The listing builds one solid part. Answer for the finished solid, in the listing's coordinates (mm). A direction names the side the tool comes from. Coordinates: 2 decimals unless noted, no trailing zeros. Write each loop counter-clockwise with the first axis right and the second up, starting at its lowest first coordinate (ties: lowest second). Pieces come first, ordered by that corner, then holes.
from build123d import *

# Parameters (mm, degrees)
SKETCH1_W           = 106
SKETCH1_H           = 48
SKETCH1_R           = 2.5
BOSS_EXTRUDE3_DEPTH = 3
BOSS_EXTRUDE4_DEPTH = 24


with BuildPart() as part:
    # Sketch1 → Boss-Extrude3 (new body)
    with BuildSketch(Plane(origin=(0, 0, 0), x_dir=(1, 0, 0), z_dir=(0, 1, 0))):
        with Locations((-8.19327026, 12.513208654)):
            Rectangle(SKETCH1_W, SKETCH1_H)
        with Locations(Location((-54.723551999, 30.013208654, 0), (0, 0, 270))):
            Circle(SKETCH1_R, mode=Mode.SUBTRACT)
        with Locations(Location((-54.690171501, -4.986791346, 0), (0, 0, 270))):
            Circle(SKETCH1_R, mode=Mode.SUBTRACT)
        with Locations(Location((38.31560417, 30.013208654, 0), (0, 0, 270))):
            Circle(SKETCH1_R, mode=Mode.SUBTRACT)
        with Locations(Location((38.297946807, -4.986791346, 0), (0, 0, 270))):
            Circle(SKETCH1_R, mode=Mode.SUBTRACT)
    extrude(amount=BOSS_EXTRUDE3_DEPTH)

    # Sketch3 → Boss-Extrude4 (add)
    with BuildSketch(Plane(origin=(0, 3, 0), x_dir=(1, 0, 0), z_dir=(0, 1, 0))):
        Polygon((-44.19327026, 32.513208654), (-44.19327026, -7.486791346), (-21.19327026, -7.486791346), (-21.19327026, -11.486791346), (-48.19327026, -11.486791346), (-48.19327026, 36.513208654), (31.80672974, 36.513208654), (31.80672974, -11.486791346), (4.80672974, -11.486791346), (4.80672974, -7.486791346), (27.80672974, -7.486791346), (27.80672974, 32.513208654), align=None)
    extrude(amount=BOSS_EXTRUDE4_DEPTH)


solid = part.part
1. Section C-C on x = -11.5 is taken. Give the vertices of the cut face in (y, z).
Results found:
outline: (0, -36.51) - (27, -36.51) - (27, -32.51) - (3, -32.51) - (3, 11.49) - (0, 11.49) - close
2. For a pull along X with two mould halves and no side action, classify faces 6 (the flat face through (-9, 1, 11.487)), 7 (the flat face through (-61.193, 1, -12)), 8 (the flat face through (-9, 3, -11)) as pulls with the +X half, pulls with the -X half, needs draft (parallel to the pull), parting line crosses it, or undercut.
Results found:
face 6: needs draft
face 7: pulls with the -X half
face 8: undercut
3. Find the intervals of material crossed by L1, parallel to X at y = 12, z = -15.5; L2, parallel to Z at x = -24, y = 22; L3, parallel to Y at x = 34, z = -5.5, in increasing order.
Results found:
L1: x = -48.19 to -44.19, 27.81 to 31.81
L2: z = -36.51 to -32.51, 7.49 to 11.49
L3: y = 0 to 3
4. Section B-B on y = 21 is taken. Give the vertices of the cut face in (x, z).
Results found:
outline: (-48.19, -36.51) - (31.81, -36.51) - (31.81, 11.49) - (4.81, 11.49) - (4.81, 7.49) - (27.81, 7.49) - (27.81, -32.51) - (-44.19, -32.51) - (-44.19, 7.49) - (-21.19, 7.49) - (-21.19, 11.49) - (-48.19, 11.49) - close
5. Section D-D on x = 7 is taken. Give the vertices of the cut face in (y, z), then the cut area to 3 significant figures.
Results found:
outline: (0, -36.51) - (27, -36.51) - (27, -32.51) - (3, -32.51) - (3, 7.49) - (27, 7.49) - (27, 11.49) - (0, 11.49) - close
area: 336 mm2
6. Flat-ended cylindrical pins translate along their axes: P1, Ø12, axis at y = 19, z = -10, coming from the -X side; P2, Ø4, axis at x = -56, z = -24, coming from the +Y side; P3, Ø7, axis at y = 17.5, z = -17, coming from the +X side. Find the tip coordinate at first contact, or state that the pin passes through.
Results found:
P1: stops at x = -48.19
P2: stops at y = 3
P3: stops at x = 31.81
7. Section A-A on z = -26.5 is taken. Give the vertices of the cut face in (x, y).
Results found:
outline: (-61.19, 0) - (44.81, 0) - (44.81, 3) - (31.81, 3) - (31.81, 27) - (27.81, 27) - (27.81, 3) - (-44.19, 3) - (-44.19, 27) - (-48.19, 27) - (-48.19, 3) - (-61.19, 3) - close
8. A tool of negligible diameter and unlimited length cuts with its end or side. For faces 1 (the flat face through (16, 15, 7.487)), 2 (the flat face through (-55, 3, -13)), 3 (the flat face through (38, 3, -13)), 4 (the flat face through (-9, 0, -13)), 5 (the flat face through (4.807, 15, 10)), from which of +Z, -Z, +X, -X, +Y, -Y can it reach the whole face along a straight path? Write none if from no direction.
Results found:
face 1: +Y
face 2: +Z, -Z, -X, +Y
face 3: +Z, -Z, +X, +Y
face 4: +Z, -Z, +X, -X, -Y
face 5: +Z, +Y
